Input: part model. Units: mm. Frame: model coordinates. A direction names the side the tool comes from. Coordinates: 2 decimals unless noted, no trailing zeros. Order: outer loops, then holes, each group sorted by start corner. A loop starts at its lowest first (then second) coordinate and runs counter-clockwise, first axis right, second up. Notation, with made-up numbers: (72.5, 55.5) -> (108.5, 55.5) arc R16 ccw to (108.5, 73.5) -> close; hole circle Ø5 at (81.5, -28). An arc over 180 degrees is marked (long way). Use CSV: the item, a comma, the result in double quotes. Start each with the question number.
```python
from build123d import *

# Parameters (mm, degrees)
SKETCH1_R           = 8.939106544
BOSS_EXTRUDE1_DEPTH = 10


with BuildPart() as part:
    # Sketch1 → Boss-Extrude1 (new body)
    with BuildSketch(Plane.XY):
        with BuildLine():
            Line((29.527184843, 92.970730655), (-29.527184843, 92.970730655))
            Line((-29.527184843, 92.970730655), (-29.527184843, 71.764892873))
            ThreePointArc((-29.527184843, 71.764892873), (-18.816760055, 61.051662511), (-14.896597759, 46.418862659))
            Line((-14.896597759, 46.418862659), (-14.896597759, -46.418862659))
            ThreePointArc((-14.896597759, -46.418862659), (-18.816760055, -61.051662511), (-29.527184843, -71.764892873))
            Line((-29.527184843, -71.764892873), (-29.527184843, -92.970730655))
            Line((-29.527184843, -92.970730655), (29.527184843, -92.970730655))
            Line((29.527184843, -92.970730655), (29.527184843, -71.764892873))
            ThreePointArc((29.527184843, -71.764892873), (18.816760055, -61.051662511), (14.896597759, -46.418862659))
            Line((14.896597759, -46.418862659), (14.896597759, 46.418862659))
            ThreePointArc((14.896597759, 46.418862659), (18.816760055, 61.051662511), (29.527184843, 71.764892873))
            Line((29.527184843, 71.764892873), (29.527184843, 92.970730655))
        make_face()
        Circle(SKETCH1_R, mode=Mode.SUBTRACT)
    extrude(amount=BOSS_EXTRUDE1_DEPTH)


solid = part.part
```
1. Pull-direction query (Y, two-part tool) for faces 4 (the face through (-14.897, 1, 5)), 5 (the face through (29.527, -83, 5)), 6 (the face through (0, -92.971, 5)); classes: released by +Y, released by -Y, zero draft, split by the parting line, or undercut.
2. Contact query for flat-ended pins moving along their axis: P1, Ø2, axis at x = 16, y = -69, coming from the -Z side; P2, Ø1, axis at y = 61, z = 6, coming from the -X side; P3, Ø5, axis at y = 6.5, z = 6, coming from the -X side; P4, Ø5, axis at y = -13.5, z = 5.5, coming from the +X side. Output: stop coordinate, or through.
3. Section A-A on z = 3.5. Return loops of the section in (x, y), then the cut area to 3 significant figures.
4. Section D-D on y = 44. Return loops of the section in (x, z), then the cut area to 3 significant figures.
5. Section B-B on y = 0. Return loops of the section in (x, z), then the cut area to 3 significant figures.
6. Section C-C on x = 0. Return loops of the section in (y, z), then the cut area to 3 significant figures.
7. Access query for faces 1 (the face through (-18.925, 61.237, 4.93)), 2 (the face through (14.897, -1, 5)), 3 (the face through (-14, 1, 10)). Directions: +Z, -Z, +X, -X, +Y, -Y. A direction counts if a zero-diameter tool reaches every point of the face in a straight line with its end or side. Return the directions, or none.
8. Material intervals for line 1 along Y through (x, z) = (0, 5.5); line 2 along X through (y, z) = (29.5, 4.25); line 3 along Y through (x, z) = (-22.5, 7.5), sorted ascending.
Values follow:
1,face 4,"undercut"
1,face 5,"zero draft"
1,face 6,"released by -Y"
2,P1,"stops at z = 0"
2,P2,"stops at x = -19.08"
2,P3,"stops at x = -14.9"
2,P4,"stops at x = 14.9"
3,outline,"(-29.53, -92.97) -> (29.53, -92.97) -> (29.53, -71.76) arc R29.27 cw to (14.9, -46.42) -> (14.9, 46.42) arc R29.27 cw to (29.53, 71.76) -> (29.53, 92.97) -> (-29.53, 92.97) -> (-29.53, 71.76) arc R29.27 cw to (-14.9, 46.42) -> (-14.9, -46.42) arc R29.27 cw to (-29.53, -71.76) -> close; hole circle Ø17.88 at (0, 0)"
3,area,"6,960 mm2"
4,outline,"(-14.9, 0) -> (14.9, 0) -> (14.9, 10) -> (-14.9, 10) -> close"
4,area,"298 mm2"
5,outline,"(-14.9, 0) -> (-8.94, 0) -> (-8.94, 10) -> (-14.9, 10) -> close; (8.94, 0) -> (14.9, 0) -> (14.9, 10) -> (8.94, 10) -> close"
5,area,"119 mm2"
6,outline,"(-92.97, 0) -> (-8.94, 0) -> (-8.94, 10) -> (-92.97, 10) -> close; (8.94, 0) -> (92.97, 0) -> (92.97, 10) -> (8.94, 10) -> close"
6,area,"1,680 mm2"
7,face 1,"+Z, -Z, -X"
7,face 2,"+Z, -Z, +X"
7,face 3,"+Z, +X, -X, +Y, -Y"
8,line 1,"y = -92.97 to -8.94, 8.94 to 92.97"
8,line 2,"x = -14.9 to 14.9"
8,line 3,"y = -92.97 to -66.1, 66.1 to 92.97"
